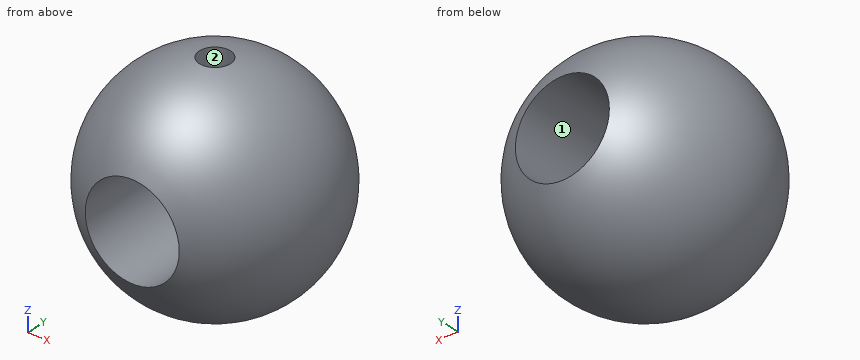
```python
from build123d import *

# Parameters (mm, degrees)
CORTAR_EXTRUIR1_DEPTH      = 17.454482672
CORTAR_EXTRUIR1_DEPTH_BACK = 10
CROQUIS2_R                 = 4
CROQUIS4_W                 = 1.3208
CROQUIS4_H                 = 9.5


with BuildPart() as part:
    # Croquis1 → Revolución1 (revolve)
    with BuildSketch(Plane.XY):
        with BuildLine():
            Line((0, -9.5), (0, 9.5))
            ThreePointArc((0, 9.5), (9.5, 0), (0, -9.5))
        make_face()
    revolve(axis=Axis((0, -9.5, 0), (0, 1, 0)))

    # Croquis2 → Cortar-Extruir1 (cut, two sides: drawn at the far end of the back side and taken through both)
    with BuildSketch(Plane(origin=(0, 0, 0), x_dir=(1, 0, 0), z_dir=(0, 1, 0)).offset(-CORTAR_EXTRUIR1_DEPTH_BACK)):
        with Locations(Location((0, 0, 0), (0, 0, 180))):
            Circle(CROQUIS2_R)
    extrude(amount=CORTAR_EXTRUIR1_DEPTH + CORTAR_EXTRUIR1_DEPTH_BACK, mode=Mode.SUBTRACT)

    # Croquis4 → Diámetro de taladro #37 (0.104)1 (revolve, cut)
    with BuildSketch(Plane.YZ):
        with Locations((0.6604, 4.75)):
            Rectangle(CROQUIS4_W, CROQUIS4_H)
    revolve(axis=Axis((0, 0, -6.35), (0, 0, 1)), mode=Mode.SUBTRACT)


solid = part.part
```
Geometry: final body of the model. Coordinates: model frame, mm. Face numbers are marked on the shaded views. A direction names the side the tool comes from. Round coordinates to 2 decimals unless told otherwise and drop trailing zeros. Loops run counter-clockwise (first coordinate to the right, second up) from the corner with the lowest first, then second, coordinate; pieces in that order, holes last. Notation, with made-up numbers: (26, -22.5) -> (78, -22.5) arc R18 cw to (78, 9.5) -> close; hole circle Ø2 at (-1, 38.5). An arc over 180 degrees is marked (long way). Use one line per item in the form item = value. Start each with the question number.
1) Section D-D on y = 0. Output: boundary loops of the cut face in (x, z).
2) Section B-B on z = 0. Output: boundary loops of the cut face in (x, y), then the cut area to 3 significant figures.
3) First-contact query: P1, Ø1, axis at y = 1.5, z = -6.5, coming from the +X side; P2, Ø6, axis at x = 3.5, y = -3, coming from the -Z side; P3, Ø1.5, axis at x = 5, z = -4, coming from the +Y side; P4, Ø3, axis at x = -1.5, z = 0, coming from the +Y side (1 decimal). Flat tips, straight axial feed; report the tip coordinate or a pass-through.
4) Access query for the marked faces 1 and 2. Directions: +Z, -Z, +X, -X, +Y, -Y. A direction counts if a zero-diameter tool reaches every point of the face in a straight line with its end or side. Return the directions, or none.
5) Line query: L1, parallel to Z at x = 0, y = -4; L2, parallel to X at y = 7.5, z = -0.75; L3, parallel to X at y = 0, z = 6.65. Output: solid intervals per line, ascending.
6) Section A-A on x = 0. Output: boundary loops of the cut face in (y, z), then the cut area to 3 significant figures.
7) Section C-C on y = 2. Output: boundary loops of the cut face in (x, z), then the cut area to 3 significant figures.
Response:
q1.outline = (-1.32, 3.78) -> (-1.32, 9.41) arc R9.5 ccw (long way) to (1.32, 9.41) -> (1.32, 3.78) arc R4 cw (long way) to start
q2.outline = (-4, -8.62) -> (-4, 8.62) arc R9.5 ccw to start; (4, -8.62) arc R9.5 ccw to (4, 8.62) -> close
q2.area = 136 mm^2
q3.P1 = 7.22
q3.P2 = -9.36
q3.P3 = 7.63
q3.P4 = through
q4.face_1 = +Y, -Y
q4.face_2 = +Z
q5.L1 = -8.62 to -4, 4 to 8.62
q5.L2 = -5.78 to -3.93, 3.93 to 5.78
q5.L3 = -6.78 to -1.32, 1.32 to 6.78
q6.outline = (-8.62, -4) arc R9.5 ccw to (8.62, -4) -> close; (-8.62, 4) -> (-1.32, 4) -> (-1.32, 9.41) arc R9.5 ccw to start; (1.32, 4) -> (8.62, 4) arc R9.5 ccw to (1.32, 9.41) -> close
q6.area = 122 mm^2
q7.outline = circle Ø18.57 at (0, 0); hole circle Ø8 at (0, 0)
q7.area = 221 mm^2
